Here's how the part is built. I have some questions about the finished solid (model axes, mm). A direction names the side the tool comes from. Round coordinates to 2 decimals unless told otherwise and drop trailing zeros. Write each loop counter-clockwise with the first axis right and the second up, starting at its lowest first coordinate (ties: lowest second). Pieces come first, ordered by that corner, then holes. Notation, with made-up numbers: M 57.25,-6 L 79.25,-6 A17 ccw 79.25,18 Z; hole C 50.25,22.25 d8. An arc over 180 degrees is marked long. Use one line per item in the form item = value. Start each with the question number.
Q1. We'd pull the mould along X, two halves only. Please class faces 1 (the face through (-3.906, -14, 13)), 2 (the face through (-2.62, -12.52, 40.05)), 3 (the face through (0, 0, 20)): +X half, -X half, draft (parallel to the pull), parting line (faces both ways), or undercut.
Q2. I want a section at A-A on z = 6. List the corners of the cut face in (x, y) for me.
Q3. I'm going to push flat-ended pins straight in: pin 1 Ø8 at (y, z) = (-21.5, 36) entering from -X; pin 2 Ø12 at (x, y) = (14.5, -9) entering from +Z; pin 3 Ø4.5 at (y, z) = (-11, 18) entering from +X; pin 4 Ø10 at (y, z) = (-10.5, 12) entering from -X. Where does each tip first touch, or does it pass through?
Q4. I want a section at C-C on z = 21. List the corners of the cut face in (x, y) for me, and give its area (3 significant figures).
Q5. I need wall thicknesses on line 1 along Y through (x, z) = (0.5, 16); line 2 along X through (y, z) = (-19.75, 24); line 3 along Z through (x, y) = (0, -7). Which ranges of each line are inside material? Lowest first, please. Write a range as from..to.
Q6. For faces 4 (the face through (0, -14, 25.4)), 5 (the face through (0, -25.4, 20)), which set-ups out of +Z, -Z, +X, -X, +Y, -Y let a thin tool reach every point of the face, with its end or its side?
Q7. I want a section at B-B on x = 0. List the corners of the cut face in (y, z) for me.
Q8. I want a section at D-D on y = -2.5. List the corners of the cut face in (x, z) for me, and give its area (3 significant figures).
```python
from build123d import *

# Parameters (mm, degrees)
F1_R     = 20.111013
F2_DEPTH = 25.4
F3_W     = 7.812914
F3_H     = 15.625822
F4_DEPTH = 25.4


with BuildPart() as f2:
    # F1 (on Front) → F2 (new body)
    with BuildSketch(Plane.XZ):
        with Locations((0, 20.111013)):
            Circle(F1_R)
    extrude(amount=F2_DEPTH)

    # F3 (on Top) → F4 (cut)
    with BuildSketch(Plane.XY):
        with Locations((0, -13.889621)):
            Rectangle(F3_W, F3_H)
    extrude(amount=F4_DEPTH, mode=Mode.SUBTRACT)


solid = f2.part
```
Reported:
q1.face_1 = undercut
q1.face_2 = parting line
q1.face_3 = draft
q2.outline = M -14.33,-25.4 L 14.33,-25.4 L 14.33,0 L -14.33,0 Z; hole M -3.91,-21.7 L 3.91,-21.7 L 3.91,-6.08 L -3.91,-6.08 Z
q3.pin_1 = -16.22
q3.pin_2 = 38.34
q3.pin_3 = 20.11
q3.pin_4 = -19.87
q4.outline = M -20.09,-25.4 L 20.09,-25.4 L 20.09,0 L -20.09,0 Z; hole M -3.91,-21.7 L 3.91,-21.7 L 3.91,-6.08 L -3.91,-6.08 Z
q4.area = 899 mm^2
q5.line_1 = -25.4..-21.7, -6.08..0
q5.line_2 = -19.73..-3.91, 3.91..19.73
q5.line_3 = 25.4..40.22
q6.face_4 = -Z
q6.face_5 = +Z, -Z, +X, -X, -Y
q7.outline = M -25.4,0 L -21.7,0 L -21.7,25.4 L -6.08,25.4 L -6.08,0 L 0,0 L 0,40.22 L -25.4,40.22 Z
q8.outline = C 0,20.11 d40.22
q8.area = 1,270 mm^2
